Part model, mm, in its own coordinate system. Round coordinates to 2 decimals unless told otherwise and drop trailing zeros. Write each loop counter-clockwise with the first axis right and the second up, starting at its lowest first coordinate (ties: lowest second). Pieces come first, ordered by that corner, then holes. Notation, with made-up numbers: (-35.75, 52) -> (-2.75, 52) arc R12 cw to (-2.75, 71) -> close; hole circle Ø9 at (31, -28). An arc over 180 degrees is marked (long way). Use CSV: the item, a comma, the result in double quotes. Start each with the question number.
(1) Saw through at B-B (x = 289). Give the cut face in (y, z), plus the area to 3 significant figures.
(2) Drop flat-ended pins along their axis: pin 1 (8 mm diameter, centred on x = 170, y = 345, fed in from -Z); pin 2 (3 mm diameter, centred on y = 342, z = 4.5, fed in from +X); pin 3 (1 mm diameter, centred on x = 138.5, z = 3.5, fed in from -Y); pin 4 (3 mm diameter, centred on x = 321, z = 4.5, fed in from +Y). Give the stop position or say it passes through.
(3) Probe line 1 (X direction, y = 275, z = 5.25); line 2 (Y direction, x = 10, z = 4.5); line 3 (X direction, y = 345, z = 4.5). List the from-to ranges inside material, lowest first. Write a range as [from, to].
(4) Saw through at A-A (z = 2.25). Give the cut face in (x, y).
```python
from build123d import *

# Parameters (mm, degrees)
SKETCH1_R           = 3
BOSS_EXTRUDE1_DEPTH = 6.35


with BuildPart() as part:
    # Sketch1 → Boss-Extrude1 (new body)
    with BuildSketch(Plane.XY):
        Polygon((0, 333), (0, 0), (127, 0), (127, 50), (213, 50), (213, 0), (340, 0), (340, 333), (284, 333), (284, 355), (56, 355), (56, 333), align=None)
        with Locations((40, 10)):
            Circle(SKETCH1_R, mode=Mode.SUBTRACT)
        with Locations((10, 80)):
            Circle(SKETCH1_R, mode=Mode.SUBTRACT)
        with Locations((300, 10)):
            Circle(SKETCH1_R, mode=Mode.SUBTRACT)
        with Locations((314.023307373, 80)):
            Circle(SKETCH1_R, mode=Mode.SUBTRACT)
        with Locations((10, 275)):
            Circle(SKETCH1_R, mode=Mode.SUBTRACT)
        with Locations((170, 345)):
            Circle(SKETCH1_R, mode=Mode.SUBTRACT)
        with Locations((317.023307373, 275)):
            Circle(SKETCH1_R, mode=Mode.SUBTRACT)
    extrude(amount=BOSS_EXTRUDE1_DEPTH)


solid = part.part
```
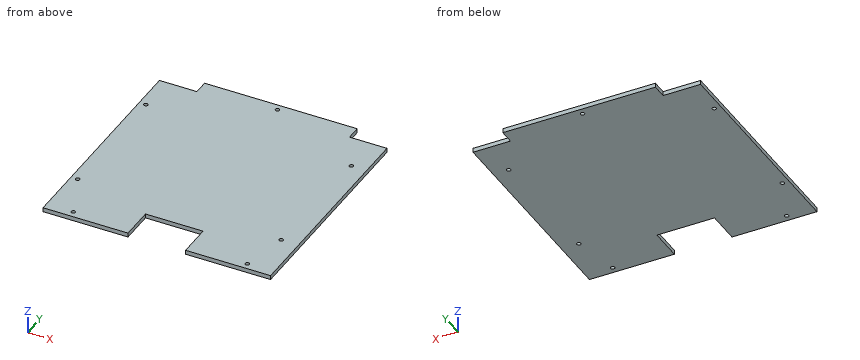
Answers:
1,outline,"(0, 0) -> (333, 0) -> (333, 6.35) -> (0, 6.35) -> close"
1,area,"2,110 mm²"
2,pin 1,"stops at z = 0"
2,pin 2,"stops at x = 284"
2,pin 3,"stops at y = 50"
2,pin 4,"stops at y = 333"
3,line 1,"x = [0, 7], [13, 314.02], [320.02, 340]"
3,line 2,"y = [0, 77], [83, 272], [278, 333]"
3,line 3,"x = [56, 167], [173, 284]"
4,outline,"(0, 0) -> (127, 0) -> (127, 50) -> (213, 50) -> (213, 0) -> (340, 0) -> (340, 333) -> (284, 333) -> (284, 355) -> (56, 355) -> (56, 333) -> (0, 333) -> close; hole circle Ø6 at (10, 80); hole circle Ø6 at (10, 275); hole circle Ø6 at (40, 10); hole circle Ø6 at (170, 345); hole circle Ø6 at (300, 10); hole circle Ø6 at (314.02, 80); hole circle Ø6 at (317.02, 275)"
